from build123d import *

# Parameters (mm, degrees)
SKETCH_1_R          = 150
EXTRUDE_1_DEPTH     = 100
SKETCH_2_W          = 200
SKETCH_2_H          = 300
EXTRUDE_2_DEPTH     = 300
EXTRUDE_4_DEPTH     = 150
SKETCH_6_R          = 150
EXTRUDE_5_DEPTH     = 200
SKETCH_7_W          = 300
SKETCH_7_H          = 800
CUT_EXTRUDE_1_DEPTH = 200
FILLET_1_R          = 30
FILLET_2_R          = 30
CUT_EXTRUDE_3_DEPTH = 213.5


with BuildPart() as part:
    # 草图1 → 凸台-拉伸1 (new, symmetric)
    with BuildSketch(Plane(origin=(0, 0, 0), x_dir=(0, 0, -1), z_dir=(1, 0, 0))):
        Circle(SKETCH_1_R)
    extrude(amount=EXTRUDE_1_DEPTH, both=True)

    # 草图2 → 凸台-拉伸2 (add)
    with BuildSketch(Plane(origin=(0, 0, 0), x_dir=(1, 0, 0), z_dir=(0, 1, 0))):
        Rectangle(SKETCH_2_W, SKETCH_2_H)
    extrude(amount=EXTRUDE_2_DEPTH)

    # 草图5 → 凸台-拉伸4 (add, symmetric)
    with BuildSketch(Plane.XY):
        Polygon((-200, 300), (-200, 700), (0, 700), (200, 700), (200, 300), (0, 300), align=None)
    extrude(amount=EXTRUDE_4_DEPTH, both=True)

    # 草图6 → 凸台-拉伸5 (add, symmetric)
    with BuildSketch(Plane(origin=(0, 0, 0), x_dir=(0, 0, -1), z_dir=(1, 0, 0))):
        with Locations((0, 700)):
            Circle(SKETCH_6_R)
    extrude(amount=EXTRUDE_5_DEPTH, both=True)

    # 草图7 → 切除-拉伸1 (cut, symmetric)
    with BuildSketch(Plane.XY):
        with Locations((0, 850)):
            Rectangle(SKETCH_7_W, SKETCH_7_H)
    extrude(amount=CUT_EXTRUDE_1_DEPTH, both=True, mode=Mode.SUBTRACT)

    # 圆角1
    fillet_1_edges = [part.edges().sort_by_distance(p)[0] for p in [
        (-200, 300, 0),
    ]]
    fillet(fillet_1_edges, radius=FILLET_1_R)

    # 圆角2
    fillet_2_edges = [part.edges().sort_by_distance(p)[0] for p in [
        (200, 300, 0),
    ]]
    fillet(fillet_2_edges, radius=FILLET_2_R)

    # 草图9 → 切除-拉伸3 (cut, symmetric)
    with BuildSketch(Plane.XY):
        with BuildLine():
            Line((-150, 450), (150, 450))
            ThreePointArc((150, 450), (0, 385.920784964), (-150, 450))
        make_face()
    extrude(amount=CUT_EXTRUDE_3_DEPTH, both=True, mode=Mode.SUBTRACT)


solid = part.part
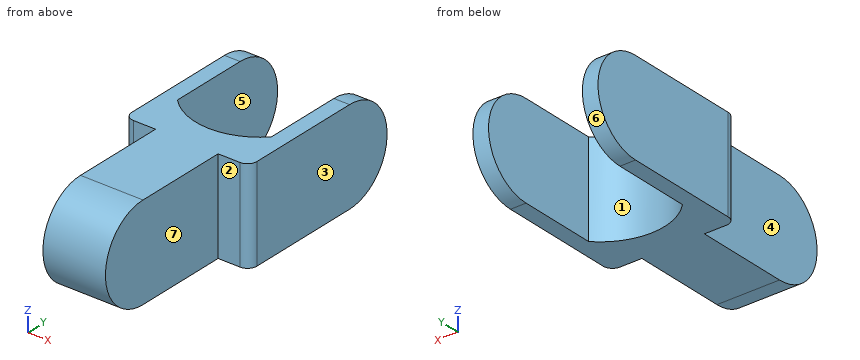
Could you check a few things on this model? Use its own coordinates, in mm. Face numbers are marked on the shaded views. A direction names the side the tool comes from. Give positions to 0.01 mm unless a question says otherwise; leave off trailing zeros. Order: outer loops, then holes, each group sorted by start corner. A loop starts at its lowest first (then second) coordinate and runs counter-clockwise, first axis right, second up. Notation, with made-up numbers: (5.5, 50) - (35.5, 50) arc R24 cw to (35.5, 75) - close; hole circle Ø7 at (68, 66.25). An arc over 180 degrees is marked (long way). One line per question, with ' | ' between items. Start each with the question number.
Item 1: For the marked faces 5, 6 and 7, which set-ups out of +Z, -Z, +X, -X, +Y, -Y let a thin tool reach every point of the face, with its end or its side?
Item 2: I want a section at D-D on x = -78. Write out the boundary of the cut face in (y, z), then the cut area to 3 significant figures.
Item 3: I want a section at B-B on z = 0. Write out the boundary of the cut face in (x, y), then the cut area to 3 significant figures.
Item 4: I'm going to push flat-ended pins straight in: pin 1 Ø2 at (x, z) = (118.5, -44.5) entering from -Y; pin 2 Ø4 at (x, z) = (-35, 27) entering from +Y; pin 3 Ø2 at (y, z) = (148, -13) entering from -X. Where does each tip first touch, or does it pass through?
Item 5: I want a section at A-A on y = 655.5. Write out the boundary of the cut face in (x, z), then the cut area to 3 significant figures.
Item 6: I want a section at C-C on y = 416. Write out the boundary of the cut face in (x, z).
Item 7: Thinking about a two-plate mould opening in X: for the marked faces 1, 2, 3 and 4, which applies, pulls with the +X half, pulls with the -X half, needs draft (parallel to the pull), parting line crosses it, or undercut?
Item 8: I need wall thicknesses on probe 1 along X at (y, z) = (789, 74); probe 2 along X at (y, z) = (-67, 27.5); probe 3 along Y at (x, z) = (-84, 56). Which ranges of each line are inside material? Lowest first, please. Write a range as [from, to].
Verdict:
1) face 5: +Z, -Z, +Y | face 6: +X, -X, +Y | face 7: +Z, -Z, +X, -Y
2) outline: (0, -150) - (401.13, -150) - (401.13, 150) - (0, 150) arc R150 ccw to start | area: 156,000 mm^2
3) outline: (-200, 330) arc R30 ccw to (-170, 300) - (-100, 300) - (-100, -150) - (100, -150) - (100, 300) - (170, 300) arc R30 ccw to (200, 330) - (200, 850) - (150, 850) - (150, 450) arc R207.6 cw to (-150, 450) - (-150, 850) - (-200, 850) - close | area: 176,000 mm^2
4) pin 1: y = 300 | pin 2: y = 389.24 | pin 3: x = -100
5) outline: (-200, -150) - (-150, -150) - (-150, 150) - (-200, 150) - close; (150, -150) - (200, -150) - (200, 150) - (150, 150) - close | area: 30,000 mm^2
6) outline: (-200, -150) - (-107.63, -150) - (-107.63, 150) - (-200, 150) - close; (107.63, -150) - (200, -150) - (200, 150) - (107.63, 150) - close
7) face 1: undercut | face 2: needs draft | face 3: pulls with the +X half | face 4: pulls with the -X half
8) probe 1: [-200, -150], [150, 200] | probe 2: [-100, 100] | probe 3: [-139.15, 403.67]
